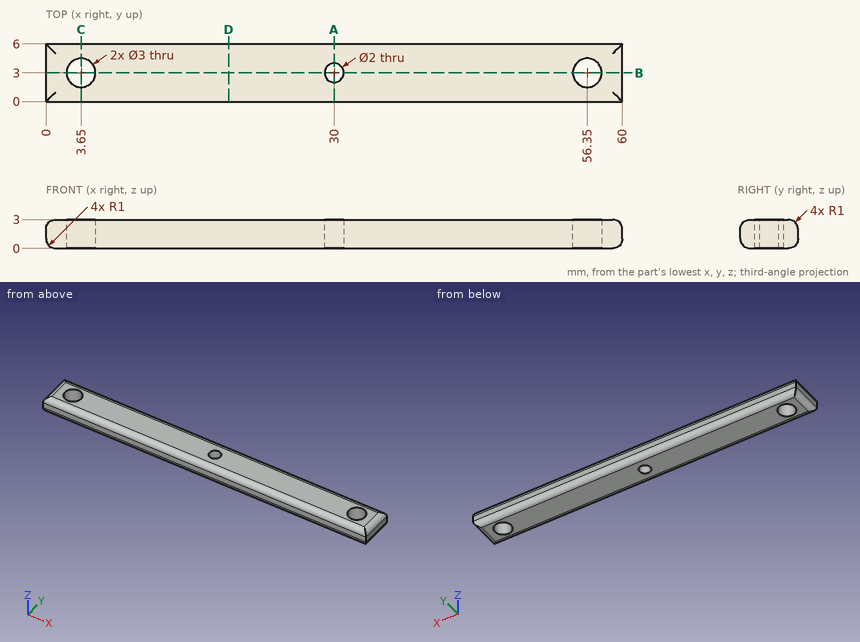
Job drawing, mm, ordinate dimensions from the low corner. One solid piece. Give positions to 0.01 mm unless a question says otherwise; leave off trailing zeros. Loops run counter-clockwise (first coordinate to the right, second up) from the corner with the lowest first, then second, coordinate; pieces in that order, holes last. Notation, with made-up numbers: M 43,50 L 76,50 A23 cw 76,75 Z; hole C 89,-24.5 d10. An arc over 180 degrees is marked long. Answer in a Markdown table with one row per item. Add a question column.
Item 1: Band-saw the part on D-D on x = 19. Give the cut face in (y, z).
Item 2: Band-saw the part on B-B on y = 3. Give the cut face in (x, z).
Item 3: Band-saw the part on A-A on x = 30. Give the cut face in (y, z).
Item 4: Band-saw the part on C-C on x = 3.65. Give the cut face in (y, z).
Item 5: Probe probe 1 along X at (y, z) = (3.55, 1.8); probe 2 along Y at (x, z) = (56.35, 1.15); probe 3 along X at (y, z) = (2.7, 1.95). List the from-to ranges inside material, lowest first.
Reply:
| question | item | result |
|---|---|---|
| 1 | outline | M 0,1 A1 ccw 1,0 L 5,0 A1 ccw 6,1 L 6,2 A1 ccw 5,3 L 1,3 A1 ccw 0,2 Z |
| 2 | outline | M 0,1 A1 ccw 1,0 L 2.15,0 L 2.15,3 L 1,3 A1 ccw 0,2 Z; M 5.15,0 L 29,0 L 29,3 L 5.15,3 Z; M 31,0 L 54.85,0 L 54.85,3 L 31,3 Z; M 57.85,0 L 59,0 A1 ccw 60,1 L 60,2 A1 ccw 59,3 L 57.85,3 Z |
| 3 | outline | M 0,1 A1 ccw 1,0 L 2,0 L 2,3 L 1,3 A1 ccw 0,2 Z; M 4,0 L 5,0 A1 ccw 6,1 L 6,2 A1 ccw 5,3 L 4,3 Z |
| 4 | outline | M 0,1 A1 ccw 1,0 L 1.5,0 L 1.5,3 L 1,3 A1 ccw 0,2 Z; M 4.5,0 L 5,0 A1 ccw 6,1 L 6,2 A1 ccw 5,3 L 4.5,3 Z |
| 5 | probe 1 | x = 0 to 2.25, 5.05 to 29.16, 30.84 to 54.95, 57.75 to 60 |
| 5 | probe 2 | y = 0 to 1.5, 4.5 to 6 |
| 5 | probe 3 | x = 0 to 2.18, 5.12 to 29.05, 30.95 to 54.88, 57.82 to 60 |
